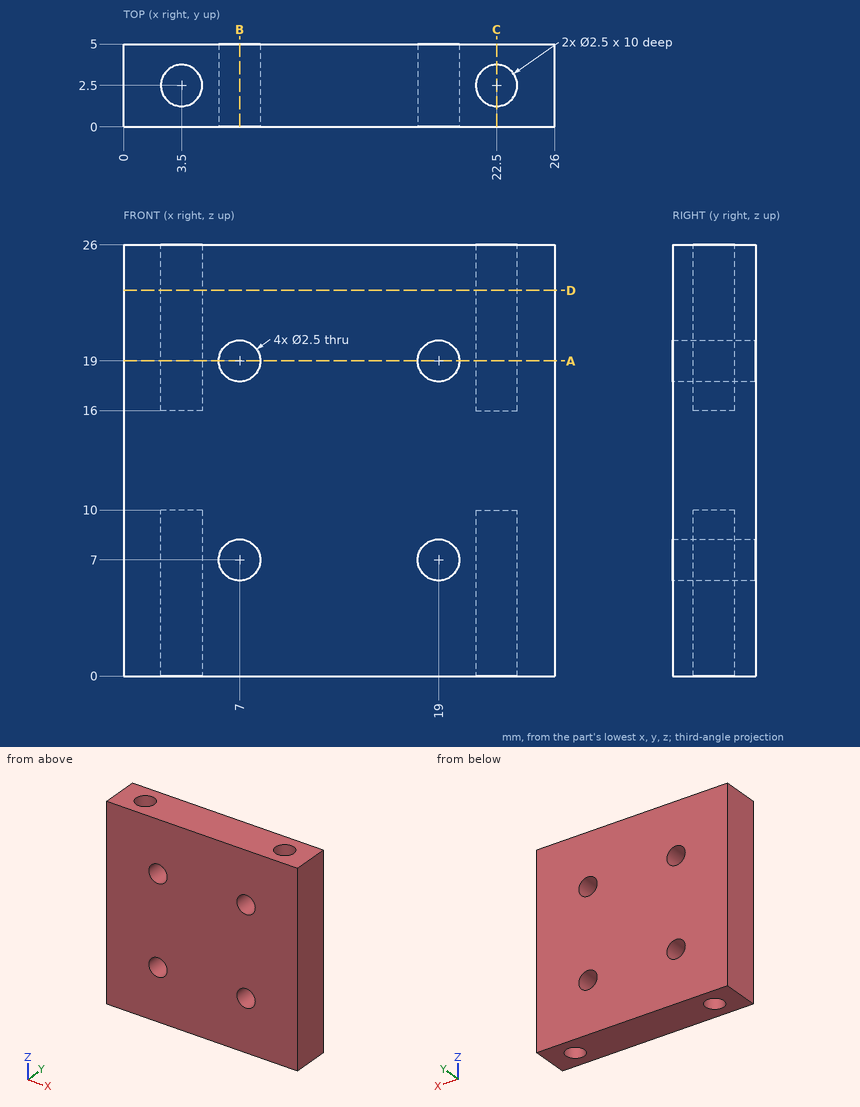
Geometry check sheet. Reference: drawing and pictorial views, mm from the part's lowest x, y, z. Give positions to 0.01 mm unless a question says otherwise; leave off trailing zeros. Order: outer loops, then holes, each group sorted by start corner. A loop starts at its lowest first (then second) coordinate and runs counter-clockwise, first axis right, second up. Notation, with made-up numbers: M -1,-30.5 L 58,-30.5 A24 cw 58,-18.5 Z; hole C 9,46.5 d4. An arc over 180 degrees is marked long. Return JSON: item names as keys, results as strings. Group by question number.
1) Section check C-C on x = 22.5. Record the cut outline in (y, z).
2) Scan lines: line 1 (X direction, y = 3.9, z = 7); line 2 (X direction, y = 1.7, z = 16.5); line 3 (Y direction, x = 3.5, z = 23.5). Record each from-to range of solid material in increasing order.
3) Section check B-B on x = 7. Record the cut outline in (y, z).
4) Section check D-D on z = 23.25. Record the cut outline in (x, y), and give its area (3 significant figures).
5) Section check A-A on z = 19. Record the cut outline in (x, y).
Answer block:
{
 "1": {"outline": "M 0,0 L 1.25,0 L 1.25,10 L 3.75,10 L 3.75,0 L 5,0 L 5,26 L 3.75,26 L 3.75,16 L 1.25,16 L 1.25,26 L 0,26 Z"},
 "2": {"line 1": "x = 0 to 5.75, 8.25 to 17.75, 20.25 to 26", "line 2": "x = 0 to 2.54, 4.46 to 21.54, 23.46 to 26", "line 3": "y = 0 to 1.25, 3.75 to 5"},
 "3": {"outline": "M 0,0 L 5,0 L 5,5.75 L 0,5.75 Z; M 0,8.25 L 5,8.25 L 5,17.75 L 0,17.75 Z; M 0,20.25 L 5,20.25 L 5,26 L 0,26 Z"},
 "4": {"outline": "M 0,0 L 26,0 L 26,5 L 0,5 Z; hole C 3.5,2.5 d2.5; hole C 22.5,2.5 d2.5", "area": "120 mm^2"},
 "5": {"outline": "M 0,0 L 5.75,0 L 5.75,5 L 0,5 Z; M 8.25,0 L 17.75,0 L 17.75,5 L 8.25,5 Z; M 20.25,0 L 26,0 L 26,5 L 20.25,5 Z; hole C 3.5,2.5 d2.5; hole C 22.5,2.5 d2.5"}
}
